For this review, take the finished solid that the model builds, in its own axes (mm). A direction names the side the tool comes from. Round coordinates to 2 decimals unless told otherwise and drop trailing zeros. Loops run counter-clockwise (first coordinate to the right, second up) from the corner with the lowest first, then second, coordinate; pieces in that order, holes last. Notation, with made-up numbers: (52.25, 89) -> (81.25, 89) arc R32 cw to (81.25, 116) -> close; hole circle Ø8 at (4, 26). An arc over 180 degrees is marked (long way). One line per question, with ' | ' between items. Start each with the question number.
1. Wall thickness on line 1 along Z through (x, y) = (0, 4.25); line 2 along Z through (x, y) = (0, -4.75); line 3 along Y through (x, z) = (13, 3): over which ranges is each line inside the solid? List them lowest first.
2. For pin 1 Ø8 at (x, z) = (1.5, -4) entering from +Y; pin 2 Ø3 at (y, z) = (-2, 7) entering from +X; pin 3 Ø1.5 at (y, z) = (-3.5, 15.5) entering from +X; pin 4 Ø1 at (y, z) = (3.5, -12.5) entering from -X, all flat-tipped, find the tip position at first contact; note any pin that passes through.
3. Draft analysis for pull direction X (two halves, no side actions). For faces 1 (the face through (-17.992, -6.563, 5.666)), 2 (the face through (-10.382, -6.993, -19.961)), 3 (the face through (-0.1, 8, 13.4)), state which applies: pulls with the +X half, pulls with the -X half, needs draft (parallel to the pull), parting line crosses it, or undercut.
4. For faces 4 (the face through (-14.985, -7.24, 0.66)), 5 (the face through (-14.985, 7.26, 0.66)), 6 (the face through (14.93, 5.55, -11.44)), list the 3-axis set-ups (+Z, -Z, +X, -X, +Y, -Y) from which the entire face can be reached by the end or side of a thin tool; tool diameter is ignored.
5. Consider section A-A (y = 1.75). Write out the cut boundary in (x, z), and give its area (3 significant figures).
```python
from build123d import *


with BuildPart() as part:
    # 草圖1 → 旋轉1 (revolve)
    with BuildSketch(Plane.XY):
        Polygon((13, 4), (13, -4), (12, -4), (12, -8), (15, -8), (15, -5.5), (18.62, -5.5), (18.62, 5.5), (15, 5.5), (15, 8), (13, 8), (13, 4.8), (13.712949133, 4.8), (13.712949133, 4), align=None)
    revolve(axis=Axis((0, 49.340027701, 0), (0, -1, 0)))

    # 草圖7 → 旋轉2 (revolve)
    with BuildSketch(Plane.XY):
        Polygon((-22.5, -6.5), (-18.62, -5.5), (-15, -5.5), (-15, -6.5), (-18.62, -6.5), (-22.5, -7.5), align=None)
    revolve_2 = revolve(axis=Axis((0, 0, 0), (0, 1, 0)))

    # 鏡射1: 旋轉2 across plane
    add(revolve_2.mirror(Plane.ZX))


solid = part.part
```
Answer block:
1) line 1: z = -18.62 to -13.71, 13.71 to 18.62 | line 2: z = -18.62 to -12, 12 to 18.62 | line 3: y = -8 to 4, 4.8 to 8
2) pin 1: passes through | pin 2: stops at x = 17.79 | pin 3: stops at x = 11.36 | pin 4: stops at x = -14.24
3) face 1: undercut | face 2: parting line crosses it | face 3: needs draft
4) face 4: -Y | face 5: +Y | face 6: none
5) outline: circle Ø37.24 at (0, 0); hole circle Ø26 at (0, 0) | area: 558 mm2
